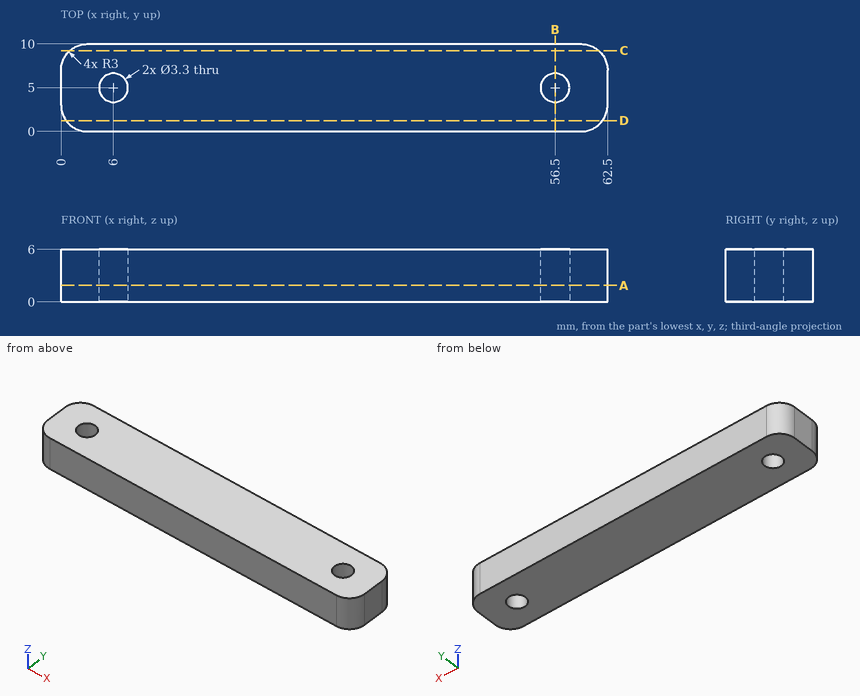
Check sheet for the drawn part. Datum: minimum x, y, z corner. Units: mm. Give positions to 0.01 mm unless a question says otherwise; leave off trailing zeros. Order: outer loops, then holes, each group sorted by start corner. A loop starts at its lowest first (then second) coordinate and runs counter-clockwise, first axis right, second up. Notation, with made-up numbers: (-0.5, 80.5) - (46.5, 80.5) arc R8 ccw to (46.5, 90.5) - close; hole circle Ø11 at (-24.5, -32.5). An arc over 180 degrees is marked (long way). Write item = value, one per line. Start each with the question number.
1) Section check B-B (x = 56.5). Enter the section's corners in (y, z).
2) Section check C-C (y = 9.25). Enter the section's corners in (x, z).
3) Section check D-D (y = 1.25). Enter the section's corners in (x, z), then the cut area to 3 significant figures.
4) Scan lines: L1, parallel to Y at x = 6, z = 4.6; L2, parallel to X at y = 6.25, z = 1.4; L3, parallel to X at y = 5.25, z = 1.2. Record each from-to range of solid material in increasing order.
5) Section check A-A (z = 1.9). Enter the section's corners in (x, y).
Geometry check:
q1.outline = (0, 0) - (3.35, 0) - (3.35, 6) - (0, 6) - close; (6.65, 0) - (10, 0) - (10, 6) - (6.65, 6) - close
q2.outline = (1.02, 0) - (61.48, 0) - (61.48, 6) - (1.02, 6) - close
q3.outline = (0.56, 0) - (61.94, 0) - (61.94, 6) - (0.56, 6) - close
q3.area = 368 mm2
q4.L1 = 0 to 3.35, 6.65 to 10
q4.L2 = 0 to 4.92, 7.08 to 55.42, 57.58 to 62.5
q4.L3 = 0 to 4.37, 7.63 to 54.87, 58.13 to 62.5
q5.outline = (0, 3) arc R3 ccw to (3, 0) - (59.5, 0) arc R3 ccw to (62.5, 3) - (62.5, 7) arc R3 ccw to (59.5, 10) - (3, 10) arc R3 ccw to (0, 7) - close; hole circle Ø3.3 at (6, 5); hole circle Ø3.3 at (56.5, 5)
